Can you work these out from the model? Positions are in its coordinate system, mm. A direction names the side the tool comes from. Round coordinates to 2 decimals unless told otherwise and drop trailing zeros. Write each loop counter-clockwise with the first axis right and the second up, starting at its lowest first coordinate (ties: lowest second). Pieces come first, ordered by that corner, then holes.
Q1. We'd pull the mould along X, two halves only. Please class faces 3 (the flat face through (0, 3, 5)), 4 (the flat face through (-27, -6, 27)), 5 (the cylindrical face through (-2.26, -6.47, 62.46)): +X half, -X half, draft (parallel to the pull), parting line (faces both ways), or undercut.
Q2. If we section it at B-B (y = 2.5): Please give me the cut outline in (x, z), plus the area to 3 significant figures.
Q3. Please list where these lines run through material, in increasing order: line 1 along Y through (x, z) = (-18.5, 52); line 2 along Z through (x, y) = (11, 5.25); line 3 along Z through (x, y) = (-4, -7.75).
Q4. For faces 1 (the flat face through (0, -6, 70)), 2 (the flat face through (0, -4, 37)), which set-ups out of +Z, -Z, +X, -X, +Y, -Y let a thin tool reach every point of the face, with its end or its side?
Q5. If we section it at D-D (x = -12): Please give me the cut outline in (y, z).
Q6. If we section it at A-A (x = -5.5): Please give me the cut outline in (y, z).
Q7. I'm going to push flat-ended pins straight in: pin 1 Ø1.5 at (x, z) = (-15, 14.5) entering from +Y; pin 2 Ø10.5 at (x, y) = (7, 2) entering from +Z. Where does each tip first touch, or does it pass through?
Q8. If we section it at C-C (z = 38): Please give me the cut outline in (x, y).
from build123d import *

# Parameters (mm, degrees)
ESQUISSE1_W             = 54
ESQUISSE1_H             = 18
BOSS_EXTRU_1_DEPTH      = 70
ESQUISSE2_W             = 89.885876072
ESQUISSE2_H             = 74.564815434
ENL_V_MAT_EXTRU_1_DEPTH = 13
M6_CLEARANCE_HOLE1_D    = 6.6
M10_CLEARANCE_HOLE1_D   = 11


with BuildPart() as part:
    # Esquisse1 → Boss.-Extru.1 (new body)
    with BuildSketch(Plane.XY):
        Rectangle(ESQUISSE1_W, ESQUISSE1_H)
    extrude(amount=BOSS_EXTRU_1_DEPTH)

    # Esquisse2 → Enlèv. mat.-Extru.1 (cut)
    with BuildSketch(Plane(origin=(0, 9, 0), x_dir=(1, 0, 0), z_dir=(0, 1, 0))):
        with Locations((-2.437014962, -42.282407717)):
            Rectangle(ESQUISSE2_W, ESQUISSE2_H)
    extrude(amount=-ENL_V_MAT_EXTRU_1_DEPTH, mode=Mode.SUBTRACT)

    # M6 Clearance Hole1 (through all)
    with Locations(Plane.XY.offset(5)):
        with Locations((19.211630693, 1.144746785), (-17.782403657, 1.144746785)):
            Hole(M6_CLEARANCE_HOLE1_D / 2)

    # M10 Clearance Hole1 (through all)
    with Locations(Plane(origin=(0, -9, 0), x_dir=(-1, 0, 0), z_dir=(0, -1, 0))):
        with Locations((1.06980506, -57.092210499)):
            Hole(M10_CLEARANCE_HOLE1_D / 2)


solid = part.part
A:
1. face 3: draft
1. face 4: -X half
1. face 5: undercut
2. outline: (-27, 0) - (-20.79, 0) - (-20.79, 5) - (-27, 5) - close; (-14.77, 0) - (16.2, 0) - (16.2, 5) - (-14.77, 5) - close; (22.22, 0) - (27, 0) - (27, 5) - (22.22, 5) - close
2. area: 210 mm2
3. line 1: y = -9 to -4
3. line 2: z = 0 to 5
3. line 3: z = 0 to 52.44, 61.75 to 70
4. face 1: +Z, +X, -X, +Y, -Y
4. face 2: +Z, +X, -X, +Y
5. outline: (-9, 0) - (9, 0) - (9, 5) - (-4, 5) - (-4, 70) - (-9, 70) - close
6. outline: (-9, 0) - (9, 0) - (9, 5) - (-4, 5) - (-4, 53.83) - (-9, 53.83) - close; (-9, 60.35) - (-4, 60.35) - (-4, 70) - (-9, 70) - close
7. pin 1: stops at y = -4
7. pin 2: stops at z = 5
8. outline: (-27, -9) - (27, -9) - (27, -4) - (-27, -4) - close
